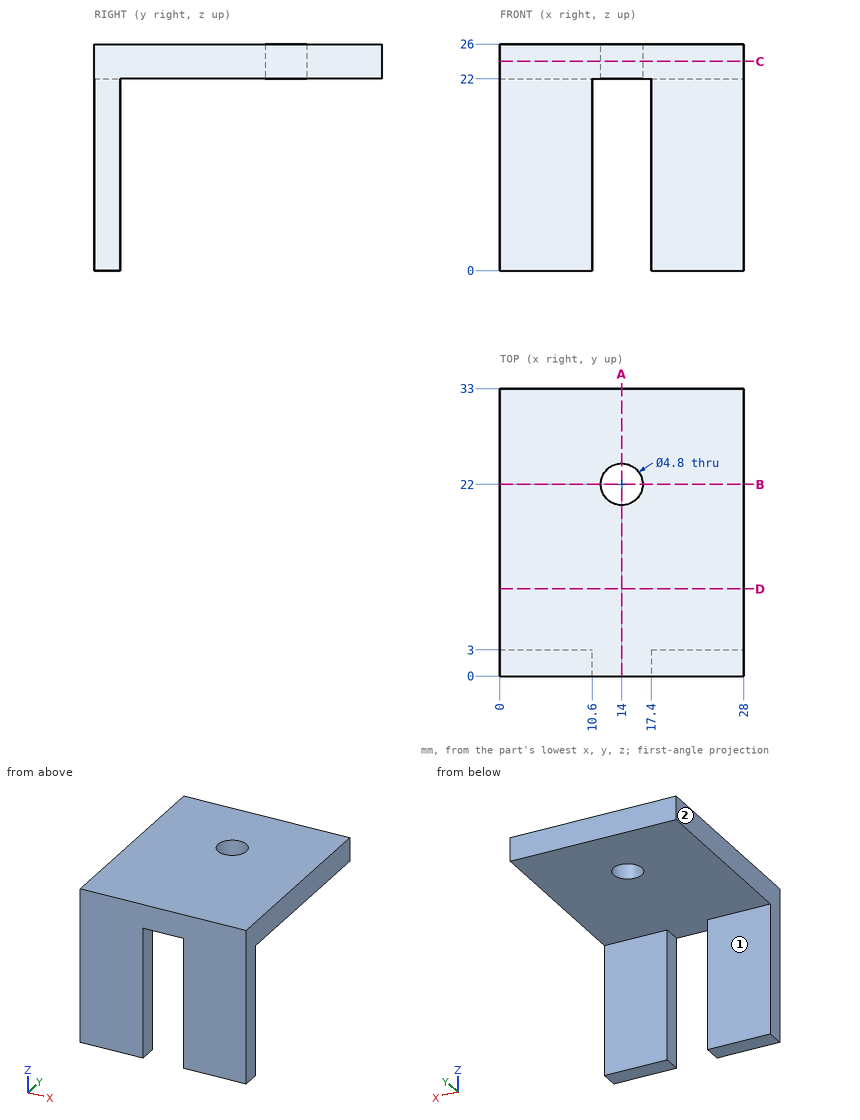
Check sheet for the drawn part. Datum: minimum x, y, z corner. Units: mm. A direction names the side the tool comes from. Give positions to 0.01 mm unless a question says otherwise; leave off trailing zeros. Write each loop counter-clockwise with the first axis right and the second up, starting at its lowest first coordinate (ties: lowest second). Pieces come first, ordered by that corner, then holes.
(1) Material ranges on line 1 (Y direction, x = 14, z = 23.3); line 2 (Y direction, x = 19.75, z = 12.5); line 3 (Z direction, x = 10, y = 7), recorded low to high.
(2) Cross-section at A-A (x = 14). Enter the section's corners in (y, z).
(3) Cross-section at B-B (y = 22). Enter the section's corners in (x, z).
(4) Access from +Z, -Z, +X, -X, +Y, -Y to the whole of each face (thin tool, end or side, straight path). Record for the marked faces 1 and 2.
(5) Cross-section at D-D (y = 10). Enter the section's corners in (x, z), plus the area to 3 significant figures.
(6) Cross-section at C-C (z = 24). Enter the section's corners in (x, y), plus the area to 3 significant figures.
(7) Gauge pin test, flat ends, axial feed: pin 1 (8.5 mm diameter, centred on x = 3.5, z = 15, fed in from +Y); pin 2 (1.5 mm diameter, centred on x = 6.5, y = 17.5, fed in from -Z). Record the tip position at first contact, or that the pin passes through.
Worked out:
1. line 1: y = 0 to 19.6, 24.4 to 33
1. line 2: y = 0 to 3
1. line 3: z = 22 to 26
2. outline: (0, 22) - (19.6, 22) - (19.6, 26) - (0, 26) - close; (24.4, 22) - (33, 22) - (33, 26) - (24.4, 26) - close
3. outline: (0, 22) - (11.6, 22) - (11.6, 26) - (0, 26) - close; (16.4, 22) - (28, 22) - (28, 26) - (16.4, 26) - close
4. face 1: -Z, +X, -X, +Y
4. face 2: +Z, -Z, -X, +Y, -Y
5. outline: (0, 22) - (28, 22) - (28, 26) - (0, 26) - close
5. area: 112 mm2
6. outline: (0, 0) - (28, 0) - (28, 33) - (0, 33) - close; hole circle Ø4.8 at (14, 22)
6. area: 906 mm2
7. pin 1: stops at y = 3
7. pin 2: stops at z = 22
